Could you check a few things on this model? Use its own coordinates, in mm. Give positions to 0.01 mm unless a question says otherwise; leave off trailing zeros. Loops run counter-clockwise (first coordinate to the right, second up) from the corner with the lowest first, then second, coordinate; pieces in that order, holes last. Notation, with made-up numbers: (-33, -35.5) -> (-17, -35.5) arc R7 cw to (-17, -30.5) -> close; hole circle Ø8 at (-1, -12). An arc over 180 degrees is marked (long way). Write item = value, one per line. Start each with the question number.
1) I want a section at B-B (y = -25). List the corners of the cut face in (x, z) for me, and give its area (3 significant figures).
2) I want a section at A-A (x = 25). List the corners of the cut face in (y, z) for me.
3) I'm going to push flat-ended pins straight in: pin 1 Ø3 at (x, y) = (-27.5, -25.5) entering from +Z; pin 2 Ø11.5 at (x, y) = (25, -25) entering from -Z; pin 3 Ø3 at (x, y) = (-25.5, -25.5) entering from -Z. Where does each tip first touch, or does it pass through?
4) I need wall thicknesses on probe 1 along X at (y, z) = (-25, -232); probe 2 along Y at (x, z) = (25, 230); probe 3 along Z at (x, y) = (-26.5, -28). Which ranges of each line are inside material? Lowest first, please. Write a range as from..to.
from build123d import *

# Parameters (mm, degrees)
F0_W     = 100
F0_H     = 500
F1_DEPTH = 50
F2_R     = 5
F3_DEPTH = 25
F4_R     = 5
F5_DEPTH = 25


with BuildPart() as f1:
    # F0 (on Front) → F1 (new body)
    with BuildSketch(Plane.XZ):
        Rectangle(F0_W, F0_H)
    extrude(amount=F1_DEPTH)

    # F2 (on face) → F3 (cut)
    with BuildSketch(Plane.XY.offset(250)):
        with Locations((-25, -25)):
            Circle(F2_R)
        with Locations((25, -25)):
            Circle(F2_R)
    extrude(amount=-F3_DEPTH, mode=Mode.SUBTRACT)

    # F4 (on face) → F5 (cut)
    with BuildSketch(Plane(origin=(0, 0, -250), x_dir=(1, 0, 0), z_dir=(0, 0, -1))):
        with Locations((25, 25)):
            Circle(F4_R)
        with Locations((-25, 25)):
            Circle(F4_R)
    extrude(amount=-F5_DEPTH, mode=Mode.SUBTRACT)


solid = f1.part
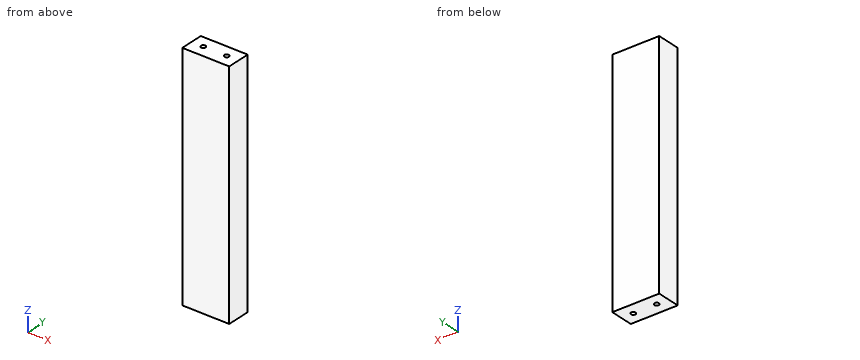
Answer list:
q1.outline = (-50, -250) -> (-30, -250) -> (-30, -225) -> (-20, -225) -> (-20, -250) -> (20, -250) -> (20, -225) -> (30, -225) -> (30, -250) -> (50, -250) -> (50, 250) -> (30, 250) -> (30, 225) -> (20, 225) -> (20, 250) -> (-20, 250) -> (-20, 225) -> (-30, 225) -> (-30, 250) -> (-50, 250) -> close
q1.area = 49,000 mm^2
q2.outline = (-50, -250) -> (-30, -250) -> (-30, -225) -> (-20, -225) -> (-20, -250) -> (0, -250) -> (0, 250) -> (-20, 250) -> (-20, 225) -> (-30, 225) -> (-30, 250) -> (-50, 250) -> close
q3.pin_1 = 225
q3.pin_2 = -250
q3.pin_3 = -225
q4.probe_1 = -50..-30, -20..20, 30..50
q4.probe_2 = -50..-30, -20..0
q4.probe_3 = -225..225
